Solid Edge part; units mm, degrees
sketch "Sketch1" plane through (0, 0, 0) normal (0, 0, 1) x (1, 0, 0)
  circle A0 centre (0, 0) radius 1.5
extrude "Protrusion1" add sketch "Sketch1" along normal blind 30
sketch "Sketch2" plane through (0, 0, 30) normal (0, 0, 1) x (1, 0, 0)
  circle A0 centre (0, 0) radius 3
extrude "ExtrudedProtrusion_2" add sketch "Sketch2" along normal blind 1.75
chamfer "Chamfer_1" distance 1.75 angle 45 1 edges at (-3, 0, 30)
sketch "Sketch3" plane through (0, 0, 31.75) normal (0, 0, 1) x (0, 1, 0)
  line L0 (0.8978, -1.555) -> (1.7956, 0)
  line L1 (1.7956, 0) -> (0.8978, 1.555)
  line L2 (0.8978, 1.555) -> (-0.8978, 1.555)
  line L3 (-0.8978, 1.555) -> (-1.7956, 0)
  line L4 (-1.7956, 0) -> (-0.8978, -1.555)
  line L5 (-0.8978, -1.555) -> (0.8978, -1.555)
extrude "ExtrudedCutout_1" cut sketch "Sketch3" against normal blind 1
sketch "Sketch4" plane through (0, 0, 0) normal (0, 0, -1) x (0, 1, 0)
  circle A0 centre (0, 0) radius 1.9215
extrude "ExtrudedCutout_2" cut sketch "Sketch4" against normal blind 13.75
properties material "Iron, grey cast type 20"
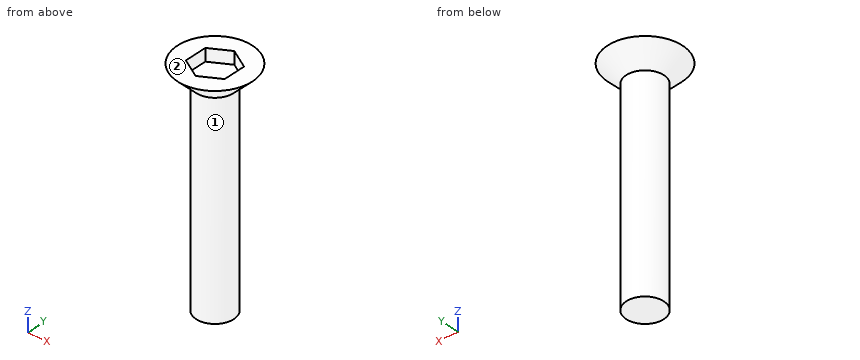
Verification items for the finished model (mm, model axes). Face numbers are marked on the shaded views. A direction names the side the tool comes from. Give positions to 0.01 mm unless a question says otherwise; leave off trailing zeros. Loops run counter-clockwise (first coordinate to the right, second up) from the corner with the lowest first, then second, coordinate; pieces in that order, holes last.
1. Go/stop test with flat-tipped pins: pin 1 Ø1 at (x, z) = (0, 20.5) entering from +Y; pin 2 Ø2 at (x, y) = (2, 0) entering from -Z; pin 3 Ø1.6 at (x, y) = (0, 0.5) entering from +Z; pin 4 Ø1.5 at (y, z) = (0.5, 23) entering from -X. Record where each tip stops, or that it passes through.
2. Section check B-B, the plane z = 29.25. Enter the section's corners in (x, y), then the cut area to 3 significant figures.
3. Section check A-A, the plane y = 0. Enter the section's corners in (x, z) (3 decimals).
4. Thickness scan on line 1 (Z direction, x = -1.15, y = 0.15); line 2 (Y direction, x = 0.05, z = 22.75); line 3 (X direction, y = 1.2, z = 24). Record the ranges inside material, lowest first.
5. Set-up check for the marked faces 1 and 2: record each of +Z, -Z, +X, -X, +Y, -Y from which the full face is reachable in a straight line by a thin tool's end or side.
Geometry says:
1. pin 1: stops at y = 1.5
1. pin 2: stops at z = 13.75
1. pin 3: stops at z = 30.75
1. pin 4: stops at x = -1.5
2. outline: circle Ø3 at (0, 0)
2. area: 7.07 mm2
3. outline: (-3, 31.75) - (-1.5, 30.25) - (-1.5, 13.75) - (1.5, 13.75) - (1.5, 30.25) - (3, 31.75) - (1.555, 31.75) - (1.555, 30.75) - (-1.555, 30.75) - (-1.555, 31.75) - close
4. line 1: z = 13.75 to 30.75
4. line 2: y = -1.5 to 1.5
4. line 3: x = -0.9 to 0.9
5. face 1: -Z
5. face 2: +Z, +X, -X, +Y, -Y
